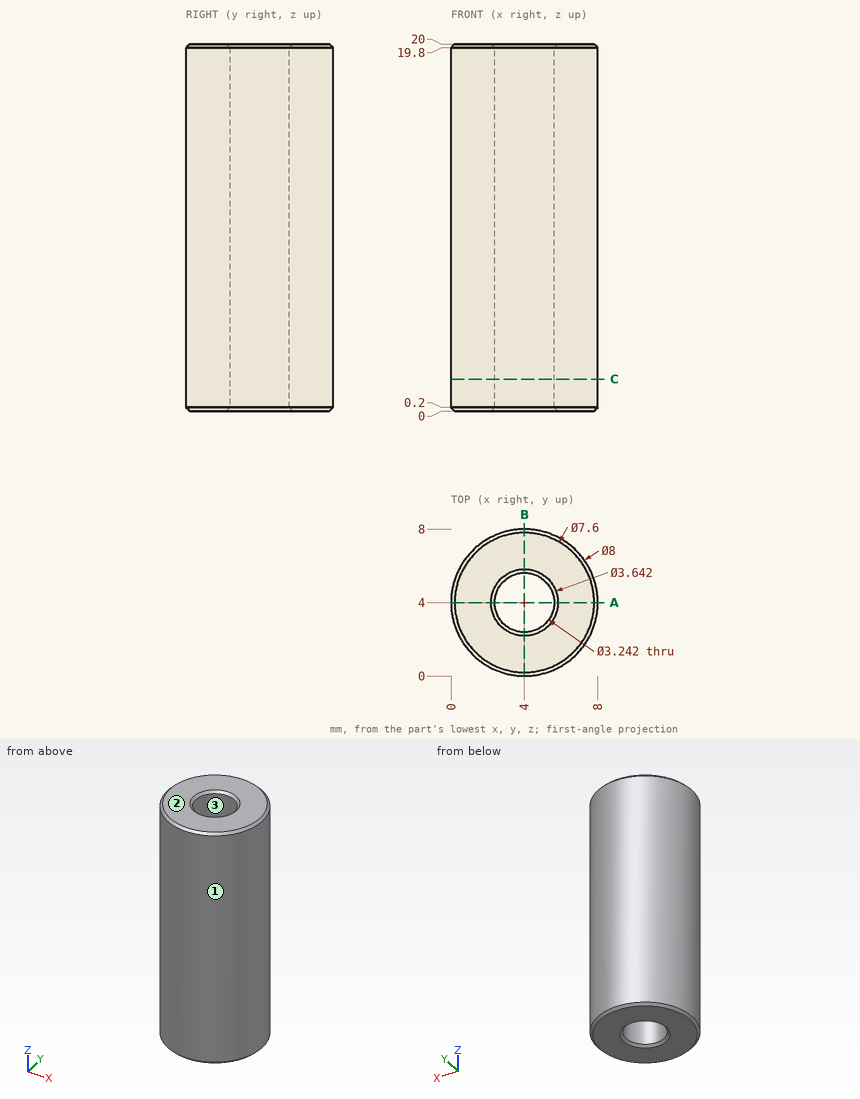
Verification items for this drawing (mm, ordinates from the low corner). Coordinates: 2 decimals unless noted, no trailing zeros. Loops run counter-clockwise (first coordinate to the right, second up) from the corner with the lowest first, then second, coordinate; pieces in that order, holes last.
Item 1: Release check for a two-part mould opening along X. For the marked faces 1, 2 and 3 record: released by +X, released by -X, zero draft, split by the parting line, or undercut.
Item 2: Sectioned sample at C-C, the plane z = 1.75. Record the boundary of the cut face in (x, y).
Item 3: Go/stop test with flat-tipped pins: pin 1 Ø1.5 at (x, z) = (6, 14.5) entering from -Y; pin 2 Ø2 at (y, z) = (1.5, 13) entering from -X; pin 3 Ø3 at (x, z) = (1.5, 12.5) entering from -Y; pin 4 Ø1.9 at (x, y) = (4, 4) entering from -Z. Record where each tip stops, or that it passes through.
Item 4: Thickness scan on line 1 (Y direction, x = 4, z = 14.5); line 2 (Y direction, x = 3.25, z = 10.25). Record the ranges inside material, lowest first.
Item 5: Sectioned sample at A-A, the plane y = 4. Record the boundary of the cut face in (x, z), then the cut area to 3 significant figures.
Check result:
1. face 1: split by the parting line
1. face 2: zero draft
1. face 3: undercut
2. outline: circle Ø8 at (4, 4); hole circle Ø3.24 at (4, 4)
3. pin 1: stops at y = 0.2
3. pin 2: stops at x = 0.29
3. pin 3: stops at y = 0.13
3. pin 4: passes through
4. line 1: y = 0 to 2.38, 5.62 to 8
4. line 2: y = 0.07 to 2.56, 5.44 to 7.93
5. outline: (0, 0.2) - (0.2, 0) - (2.18, 0) - (2.38, 0.2) - (2.38, 19.8) - (2.18, 20) - (0.2, 20) - (0, 19.8) - close; (5.62, 0.2) - (5.82, 0) - (7.8, 0) - (8, 0.2) - (8, 19.8) - (7.8, 20) - (5.82, 20) - (5.62, 19.8) - close
5. area: 95.0 mm2
